Verification items for the finished model (mm, model axes). Face numbers are marked on the shaded views. Give positions to 0.01 mm unless a question says otherwise; leave off trailing zeros. Write each loop counter-clockwise with the first axis right and the second up, starting at its lowest first coordinate (ties: lowest second). Pieces come first, ordered by that corner, then holes. Notation, with made-up numbers: M 22,20 L 54,20 A9 ccw 54,33 Z; hole C -40,-12 d4. An arc over 180 degrees is marked long. Write item = value, one per line.
from build123d import *

# Parameters (mm, degrees)
SKETCH1_R           = 1.5
SKETCH1_R_2         = 9.5
BOSS_EXTRUDE1_DEPTH = 5


with BuildPart() as part:
    # Sketch1 → Boss-Extrude1 (new body)
    with BuildSketch(Plane(origin=(0, 0, 0), x_dir=(1, 0, 0), z_dir=(0, 1, 0))):
        with BuildLine():
            Line((-11.47745757, -9.657534247), (-2.486782474, -20.342465753))
            ThreePointArc((-2.486782474, -20.342465753), (0, -21.5), (2.486782474, -20.342465753))
            Line((2.486782474, -20.342465753), (11.47745757, -9.657534247))
            ThreePointArc((11.47745757, -9.657534247), (15, 0), (11.47745757, 9.657534247))
            Line((11.47745757, 9.657534247), (2.486782474, 20.342465753))
            ThreePointArc((2.486782474, 20.342465753), (0, 21.5), (-2.486782474, 20.342465753))
            Line((-2.486782474, 20.342465753), (-11.47745757, 9.657534247))
            ThreePointArc((-11.47745757, 9.657534247), (-15, 0), (-11.47745757, -9.657534247))
        make_face()
        with Locations((0, -18.25)):
            Circle(SKETCH1_R, mode=Mode.SUBTRACT)
        Circle(SKETCH1_R_2, mode=Mode.SUBTRACT)
        with Locations((0, 18.25)):
            Circle(SKETCH1_R, mode=Mode.SUBTRACT)
    extrude(amount=BOSS_EXTRUDE1_DEPTH)


solid = part.part
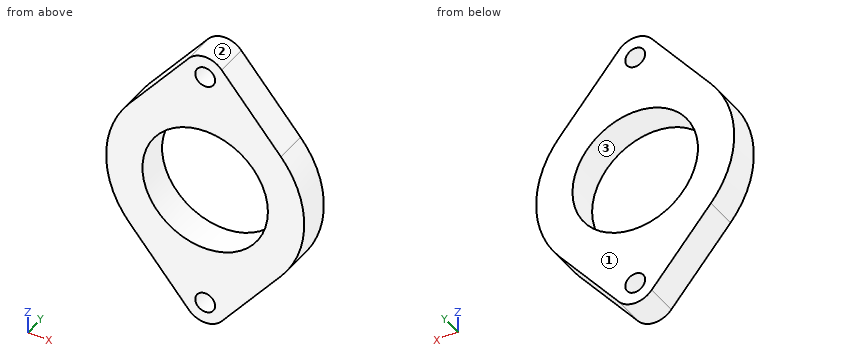
1) Cross-section at B-B on x = 0. Record the boundary of the cut face in (y, z).
From the geometry:
outline = M 0,-21.5 L 5,-21.5 L 5,-19.75 L 0,-19.75 Z; M 0,-16.75 L 5,-16.75 L 5,-9.5 L 0,-9.5 Z; M 0,9.5 L 5,9.5 L 5,16.75 L 0,16.75 Z; M 0,19.75 L 5,19.75 L 5,21.5 L 0,21.5 Z
2) Material ranges on probe 1 along Z at (x, y) = (0, 1.35); probe 2 along X at (y, z) = (1.8, 0); probe 3 along X at (y, z) = (1.1, -18.25), recorded low to high. Write a range as from..to.
From the geometry:
probe_1 = -21.5..-19.75, -16.75..-9.5, 9.5..16.75, 19.75..21.5
probe_2 = -15..-9.5, 9.5..15
probe_3 = -4.25..-1.5, 1.5..4.25
3) Depth check by flat-ended pin: P1, Ø2, axis at x = 4.5, y = 3, coming from the -Z side; P2, Ø1, axis at y = 4, z = -10.5, coming from the -X side. Enter the tip coordinate at first touch or a pass-through.
From the geometry:
P1 = -19.14
P2 = -11.19
4) Cross-section at D-D on x = 4.5. Record the boundary of the cut face in (y, z).
From the geometry:
outline = M 0,-17.95 L 5,-17.95 L 5,-8.37 L 0,-8.37 Z; M 0,8.37 L 5,8.37 L 5,17.95 L 0,17.95 Z
5) Draft check along X on the marked faces 1, 2 and 3. Enter one of: +X half, -X half, draft (parallel to the pull), parting line (faces both ways), or undercut.
From the geometry:
face_1 = draft
face_2 = parting line
face_3 = undercut
6) Cross-section at C-C on y = 1.5. Record the boundary of the cut face in (x, z), plus the area to 3 significant figures.
From the geometry:
outline = M -11.48,-9.66 L -2.49,-20.34 A3.25 ccw 2.49,-20.34 L 11.48,-9.66 A15 ccw 11.48,9.66 L 2.49,20.34 A3.25 ccw -2.49,20.34 L -11.48,9.66 A15 ccw Z; hole C 0,0 d19; hole C 0,-18.25 d3; hole C 0,18.25 d3
area = 545 mm^2
7) Cross-section at A-A on z = 0. Record the boundary of the cut face in (x, y).
From the geometry:
outline = M -15,0 L -9.5,0 L -9.5,5 L -15,5 Z; M 9.5,0 L 15,0 L 15,5 L 9.5,5 Z
